Verification items for the finished model (mm, model axes). A direction names the side the tool comes from. Give positions to 0.01 mm unless a question says otherwise; leave off trailing zeros. Order: outer loops, then holes, each group sorted by start corner. A loop starts at its lowest first (then second) coordinate and runs counter-clockwise, first axis right, second up. Notation, with made-up numbers: (18, 24.5) - (57, 24.5) arc R20 ccw to (57, 33.5) - close; hole circle Ø2 at (23, 74). An arc over 180 degrees is marked (long way). Answer as a JSON object with one key per item and string values. Group by question number.
(1) Section check A-A (y = 0.75). Record the boundary of the cut face in (x, z) (3 decimals), then the cut area to 3 significant figures.
(2) Access from +Z, -Z, +X, -X, +Y, -Y to the whole of each face (thin tool, end or side, straight path). Record for faces 5 (the face through (3, 1, -1.538)), 6 (the face through (1.3, 1.5, 0)).
(3) Section check C-C (x = 0). Record the boundary of the cut face in (y, z) (3 decimals).
(4) Depth check by flat-ended pin: pin 1 Ø1.3 at (x, z) = (0, 0) entering from -Y. Enter the tip coordinate at first touch or a pass-through.
(5) Thickness scan on line 1 (Z direction, x = 1, y = 1); line 2 (X direction, y = 0.55, z = 0.35); line 3 (X direction, y = 0.2, z = 0.8). Record the ranges inside material, lowest first.
(6) Section check B-B (z = 0). Record the boundary of the cut face in (x, y) (3 decimals).
(7) Section check D-D (x = 3.5). Record the boundary of the cut face in (y, z).
(8) Mould release check, pull along Z, two halves, no side actions. Record for faces 1 (the face through (1.09, 0.74, -0.14)), 2 (the face through (-2.174, 0.74, 0.072)), 3 (the face through (4.614, 1, 0)), 4 (the face through (3, 1, 1.538)): +Z half, -Z half, draft (parallel to the pull), parting line (faces both ways), or undercut.
```python
from build123d import *

# Parameters (mm, degrees)
SKETCH_2_R      = 1.1
EXTRUDE_1_DEPTH = 1.5


with BuildPart() as part:
    # 草图2 → 凸台-拉伸1 (new body)
    with BuildSketch(Plane(origin=(0, 0, 0), x_dir=(1, 0, 0), z_dir=(0, 1, 0))):
        with BuildLine():
            Line((1.537957249, 1.537957249), (4.613871747, 1.537957249))
            Line((4.613871747, 1.537957249), (4.613871747, -1.537957249))
            Line((4.613871747, -1.537957249), (1.537957249, -1.537957249))
            ThreePointArc((1.537957249, -1.537957249), (-2.175, 0), (1.537957249, 1.537957249))
        make_face()
        with Locations(Location((0, 0, 0), (0, 0, 270))):
            Circle(SKETCH_2_R, mode=Mode.SUBTRACT)
    extrude(amount=EXTRUDE_1_DEPTH)


solid = part.part
```
Solutions:
{
 "1": {"outline": "(1.538, -1.538) - (4.614, -1.538) - (4.614, 1.538) - (1.538, 1.538) arc R2.175 ccw (long way) to start; hole circle Ø2.2 at (0, 0)", "area": "19.2 mm2"},
 "2": {"face 5": "-Z, +X, +Y, -Y", "face 6": "+Z, -Z, +X, -X, +Y"},
 "3": {"outline": "(0, -2.175) - (1.5, -2.175) - (1.5, -1.1) - (0, -1.1) - close; (0, 1.1) - (1.5, 1.1) - (1.5, 2.175) - (0, 2.175) - close"},
 "4": {"pin 1": "passes through"},
 "5": {"line 1": "z = -1.93 to -0.46, 0.46 to 1.93", "line 2": "x = -2.15 to -1.04, 1.04 to 4.61", "line 3": "x = -2.02 to -0.75, 0.75 to 4.61"},
 "6": {"outline": "(-2.175, 0) - (-1.1, 0) - (-1.1, 1.5) - (-2.175, 1.5) - close; (1.1, 0) - (4.614, 0) - (4.614, 1.5) - (1.1, 1.5) - close"},
 "7": {"outline": "(0, -1.54) - (1.5, -1.54) - (1.5, 1.54) - (0, 1.54) - close"},
 "8": {"face 1": "undercut", "face 2": "parting line", "face 3": "draft", "face 4": "+Z half"}
}
